Source: CAD feature listing. Evaluate the final solid. Frame: model axes, mm. Face numbers are marked on the shaded views. A direction names the side the tool comes from. Round coordinates to 2 decimals unless told otherwise and drop trailing zeros. Write each loop counter-clockwise with the first axis right and the second up, starting at its lowest first coordinate (ties: lowest second). Pieces come first, ordered by that corner, then holes.
from build123d import *

# Parameters (mm, degrees)
ESQUISSE1_W                  = 60
ESQUISSE1_H                  = 40
BOSS_EXTRU_1_DEPTH           = 9
ESQUISSE2_W                  = 25
ESQUISSE2_H                  = 40
ESQUISSE2_W_2                = 5.5
ENL_V_MAT_EXTRU_1_DEPTH      = 7
ESQUISSE3_R                  = 1.55
ENL_V_MAT_EXTRU_2_DEPTH      = 36
CONG_1_R                     = 3
ESQUISSE9_R                  = 3
BOSS_EXTRU_2_DEPTH           = 3
ESQUISSE5_R                  = 1.55
ENL_V_MAT_EXTRU_4_DEPTH      = 8
ENL_V_MAT_EXTRU_4_DEPTH_BACK = 3
ESQUISSE8_W                  = 4
ESQUISSE8_H                  = 24
ENL_V_MAT_EXTRU_5_DEPTH      = 7
ESQUISSE6_W                  = 4
ESQUISSE6_H                  = 24
ENL_V_MAT_EXTRU_6_DEPTH      = 7
CONG_2_R                     = 2


with BuildPart() as part:
    # Esquisse1 → Boss.-Extru.1 (new body)
    with BuildSketch(Plane.XY):
        with Locations((30, 20)):
            Rectangle(ESQUISSE1_W, ESQUISSE1_H)
    extrude(amount=BOSS_EXTRU_1_DEPTH)

    # Esquisse2 → Enlèv. mat.-Extru.1 (cut)
    with BuildSketch(Plane(origin=(0, 0, 0), x_dir=(-1, 0, 0), z_dir=(0, 0, -1))):
        with Locations((-12.5, 20)):
            Rectangle(ESQUISSE2_W, ESQUISSE2_H)
        with Locations((-47.5, 20)):
            Rectangle(ESQUISSE2_W, ESQUISSE2_H)
        with Locations((-30, 20)):
            Rectangle(ESQUISSE2_W_2, ESQUISSE2_H)
    extrude(amount=-ENL_V_MAT_EXTRU_1_DEPTH, mode=Mode.SUBTRACT)

    # Esquisse3 → Enlèv. mat.-Extru.2 (cut, through all)
    with BuildSketch(Plane(origin=(35, 0, 0), x_dir=(0, 0, -1), z_dir=(1, 0, 0))):
        with Locations((-3.5, 15)):
            Circle(ESQUISSE3_R)
        with Locations((-3.5, 25)):
            Circle(ESQUISSE3_R)
    extrude(amount=-ENL_V_MAT_EXTRU_2_DEPTH, mode=Mode.SUBTRACT)

    # Congé1
    cong_1_edges = [part.edges().sort_by_distance(p)[0] for p in [
        (0, 40, 8),
        (60, 40, 8),
        (60, 0, 8),
        (0, 0, 8),
    ]]
    fillet(cong_1_edges, radius=CONG_1_R)

    # Esquisse9 → Boss.-Extru.2 (add)
    with BuildSketch(Plane(origin=(0, 0, 7), x_dir=(-1, 0, 0), z_dir=(0, 0, -1))):
        with Locations((-46, 35.5)):
            Circle(ESQUISSE9_R)
        with Locations((-15.5, 35.5)):
            Circle(ESQUISSE9_R)
        with Locations((-15.5, 4.75)):
            Circle(ESQUISSE9_R)
        with Locations((-46, 4.75)):
            Circle(ESQUISSE9_R)
    extrude(amount=BOSS_EXTRU_2_DEPTH)

    # Esquisse5 → Enlèv. mat.-Extru.4 (cut, two sides)
    with BuildSketch(Plane(origin=(0, 0, 7), x_dir=(-1, 0, 0), z_dir=(0, 0, -1))) as enl_v_mat_extru_4_sk:
        with Locations((-46, 35.5)):
            Circle(ESQUISSE5_R)
        with Locations((-46, 4.75)):
            Circle(ESQUISSE5_R)
        with Locations((-15.5, 4.75)):
            Circle(ESQUISSE5_R)
        with Locations((-15.5, 35.5)):
            Circle(ESQUISSE5_R)
    extrude(amount=ENL_V_MAT_EXTRU_4_DEPTH, mode=Mode.SUBTRACT)
    extrude(enl_v_mat_extru_4_sk.sketch, amount=-ENL_V_MAT_EXTRU_4_DEPTH_BACK, mode=Mode.SUBTRACT)

    # Esquisse8 → Enlèv. mat.-Extru.5 (cut)
    with BuildSketch(Plane(origin=(0, 0, 7), x_dir=(-1, 0, 0), z_dir=(0, 0, -1))):
        with Locations((-13, 20)):
            Rectangle(ESQUISSE8_W, ESQUISSE8_H)
        with Locations((-5, 20)):
            Rectangle(ESQUISSE8_W, ESQUISSE8_H)
        with Locations((-21, 20)):
            Rectangle(ESQUISSE8_W, ESQUISSE8_H)
    extrude(amount=-ENL_V_MAT_EXTRU_5_DEPTH, mode=Mode.SUBTRACT)

    # Esquisse6 → Enlèv. mat.-Extru.6 (cut)
    with BuildSketch(Plane(origin=(0, 0, 7), x_dir=(-1, 0, 0), z_dir=(0, 0, -1))):
        with Locations((-47, 20)):
            Rectangle(ESQUISSE6_W, ESQUISSE6_H)
        with Locations((-55, 20)):
            Rectangle(ESQUISSE6_W, ESQUISSE6_H)
        with Locations((-39, 20)):
            Rectangle(ESQUISSE6_W, ESQUISSE6_H)
    extrude(amount=-ENL_V_MAT_EXTRU_6_DEPTH, mode=Mode.SUBTRACT)

    # Congé2
    cong_2_edges = [part.edges().sort_by_distance(p)[0] for p in [
        (33.875, 40, 0),
        (26.125, 40, 0),
        (26.125, 0, 0),
        (33.875, 0, 0),
    ]]
    fillet(cong_2_edges, radius=CONG_2_R)


solid = part.part
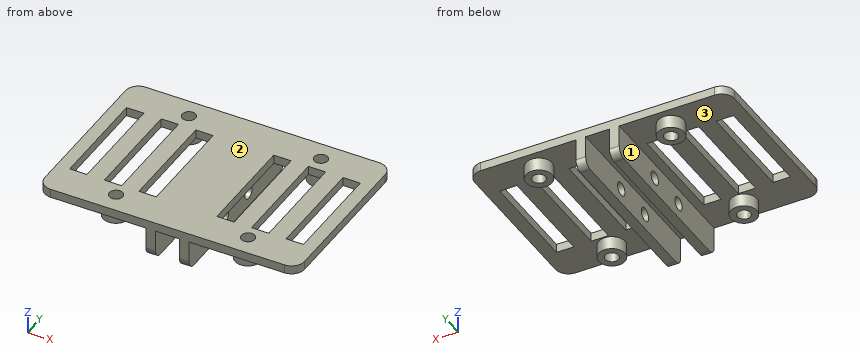
1) Material intervals for line 1 (Y direction, x = 15.5, z = 5.5); line 2 (X direction, y = 11, z = 5.25); line 3 (X direction, y = 35.5, z = 7.25), sorted ascending.
Taken from the geometry:
line 1: y = 1.75 to 3.2, 6.3 to 7.75, 32.5 to 33.95, 37.05 to 38.5
line 2: x = 25 to 27.25, 32.75 to 35
line 3: x = 0 to 13.95, 17.05 to 44.45, 47.55 to 60
2) Contact query for flat-ended pins moving along their axis: P1, Ø3.5, axis at y = 10, z = 2, coming from the -X side; P2, Ø4, axis at y = 23, z = 6.5, coming from the +X side; P3, Ø3, axis at x = 29.5, y = 21, coming from the -Z side; P4, Ø2, axis at y = 24.5, z = 4, coming from the +X side. Output: stop coordinate, or through.
Taken from the geometry:
P1: stops at x = 25
P2: stops at x = 60
P3: stops at z = 7
P4: stops at x = 35
3) Section query A-A on x = 46. Return the cut outline in (y, z).
Taken from the geometry:
outline: (0, 7) - (1.75, 7) - (1.75, 4) - (3.2, 4) - (3.2, 9) - (0, 9) - close; (6.3, 4) - (7.75, 4) - (7.75, 7) - (8, 7) - (8, 9) - (6.3, 9) - close; (32, 7) - (32.5, 7) - (32.5, 4) - (33.95, 4) - (33.95, 9) - (32, 9) - close; (37.05, 4) - (38.5, 4) - (38.5, 7) - (40, 7) - (40, 9) - (37.05, 9) - close
4) Reachability of the marked faces 1, 2 and 3 from +Z, -Z, +X, -X, +Y, -Y: full face, straight path, thin tool, end or side. Return the list, or none.
Taken from the geometry:
face 1: -Z, +Y, -Y
face 2: +Z, +X, -X, +Y, -Y
face 3: -Z
5) Section query C-C on x = 22. Return the cut outline in (y, z).
Taken from the geometry:
outline: (0, 7) - (8, 7) - (8, 9) - (0, 9) - close; (32, 7) - (40, 7) - (40, 9) - (32, 9) - close
6) Section query D-D on z = 2.75. Return the cut outline in (x, y), then the cut area to 3 significant figures.
Taken from the geometry:
outline: (25, 0) - (27.25, 0) - (27.25, 13.64) - (25, 13.64) - close; (25, 16.36) - (27.25, 16.36) - (27.25, 23.64) - (25, 23.64) - close; (25, 26.36) - (27.25, 26.36) - (27.25, 40) - (25, 40) - close; (32.75, 0) - (35, 0) - (35, 13.64) - (32.75, 13.64) - close; (32.75, 16.36) - (35, 16.36) - (35, 23.64) - (32.75, 23.64) - close; (32.75, 26.36) - (35, 26.36) - (35, 40) - (32.75, 40) - close
area: 156 mm2
7) Section query B-B on y = 4.75. Return the cut outline in (x, z), then the cut area to 4 significant figures.
Taken from the geometry:
outline: (0, 7) - (12.5, 7) - (12.5, 4) - (13.95, 4) - (13.95, 9) - (0, 9) - close; (17.05, 4) - (18.5, 4) - (18.5, 7) - (25, 7) - (25, 0) - (27.25, 0) - (27.25, 7) - (32.75, 7) - (32.75, 0) - (35, 0) - (35, 7) - (43, 7) - (43, 4) - (44.45, 4) - (44.45, 9) - (17.05, 9) - close; (47.55, 4) - (49, 4) - (49, 7) - (60, 7) - (60, 9) - (47.55, 9) - close
area: 156.5 mm2
